from build123d import *

# Parameters (mm, degrees)
F0_W     = 711.2
F0_H     = 254
F0_W_2   = 571.5
F0_H_2   = 114.3
F1_DEPTH = 19.05
F3_D     = 5.0038
F3_DEPTH = 19.05
F3_TIP   = 1.5032931827
F5_D     = 8.001
F5_DEPTH = 14.224
F5_TIP   = 2.4037429064


with BuildPart() as f1:
    # F0 (on Top) → F1 (new body)
    with BuildSketch(Plane.XY):
        Rectangle(F0_W, F0_H)
        Rectangle(F0_W_2, F0_H_2, mode=Mode.SUBTRACT)
    extrude(amount=F1_DEPTH)

    # F3
    with Locations(Plane.XY.offset(19.05)):
        with Locations((-342.9, 114.3), (-342.9, 0), (-190.5, 114.3), (190.5, 114.3), (342.9, 114.3), (342.9, 0), (342.9, -114.3), (190.5, -114.3), (-190.5, -114.3), (-342.9, -114.3), (0, 114.3), (0, -114.3)):
            Hole(F3_D / 2, depth=F3_DEPTH)
            with Locations((0, 0, -(F3_DEPTH + F3_TIP / 2))):  # 118° drill point
                Cone(0, F3_D / 2, F3_TIP, mode=Mode.SUBTRACT)

    # F5
    with Locations(Plane(origin=(0, 0, 0), x_dir=(1, 0, 0), z_dir=(0, 0, -1))):
        with Locations((-228.6, 66.675), (-228.6, -66.675), (228.6, 66.675), (228.6, -66.675)):
            Hole(F5_D / 2, depth=F5_DEPTH)
            with Locations((0, 0, -(F5_DEPTH + F5_TIP / 2))):  # 118° drill point
                Cone(0, F5_D / 2, F5_TIP, mode=Mode.SUBTRACT)


solid = f1.part
Source: CAD feature listing. Evaluate the final solid. Frame: model axes, mm. A direction names the side the tool comes from. Give positions to 0.01 mm unless a question says otherwise; leave off trailing zeros. Write each loop counter-clockwise with the first axis right and the second up, starting at its lowest first coordinate (ties: lowest second). Pieces come first, ordered by that corner, then holes. Notation, with made-up numbers: M 83.5,35.25 L 103.5,35.25 A25 ccw 103.5,47.25 Z; hole C 38,28 d11. An arc over 180 degrees is marked long. Return JSON: item names as keys, results as strings. Group by question number.
1) Cut plane B-B, the plane y = -32. Output: boundary loops of the cut face in (x, z), plus the area to 3 significant figures.
2) Material intervals for line 1 along X through (y, z) = (-114.3, 4); line 2 along Y through (x, z) = (-342.9, 4.5); line 3 along Y through (x, z) = (-59.5, 9.75), sorted ascending. Write a range as [from, to].
3) Set-up query: faces 5 (the face through (-5, 58, 0)), 6 (the face through (-4, -57.15, 9)). Return all of +Z, -Z, +X, -X, +Y, -Y with unobstructed straight access to the full face (end or side cutting, diameter ignored); none if empty.
4) Pull-direction query (Y, two-part tool) for faces 1 (the face through (285.75, -1, 9)), 2 (the face through (-355.6, -2, 9)), 3 (the face through (-4, 57.15, 9)), 4 (the face through (-5, -127, 9)); classes: pulls with the +Y half, pulls with the -Y half, needs draft (parallel to the pull), parting line crosses it, or undercut.
5) Cut plane A-A, the plane x = 59. Output: boundary loops of the cut face in (y, z), plus the area to 3 significant figures.
6) Cut plane C-C, the plane z = 5.75. Give the number of separate pieces and of enclosed holes in the cut face, plus the area to 3 significant figures.
Recorded:
{
 "1": {"outline": "M -355.6,0 L -285.75,0 L -285.75,19.05 L -355.6,19.05 Z; M 285.75,0 L 355.6,0 L 355.6,19.05 L 285.75,19.05 Z", "area": "2,660 mm²"},
 "2": {"line 1": "x = [-355.6, -345.4], [-340.4, -193], [-188, -2.5], [2.5, 188], [193, 340.4], [345.4, 355.6]", "line 2": "y = [-127, -116.8], [-111.8, -2.5], [2.5, 111.8], [116.8, 127]", "line 3": "y = [-127, -57.15], [57.15, 127]"},
 "3": {"face 5": "-Z, +X, -X, +Y, -Y", "face 6": "+Z, -Z"},
 "4": {"face 1": "undercut", "face 2": "needs draft", "face 3": "undercut", "face 4": "pulls with the -Y half"},
 "5": {"outline": "M -127,0 L -57.15,0 L -57.15,19.05 L -127,19.05 Z; M 57.15,0 L 127,0 L 127,19.05 L 57.15,19.05 Z", "area": "2,660 mm²"},
 "6": {"separate pieces": "1", "enclosed holes": "17", "area": "115,000 mm²"}
}
